Read the model definition and answer for the solid it produces. Units are mm, in the model's axes. Face numbers are marked on the shaded views. Round coordinates to 2 decimals unless told otherwise and drop trailing zeros. Write each loop counter-clockwise with the first axis right and the second up, starting at its lowest first coordinate (ties: lowest second). Pieces come first, ordered by that corner, then holes. Notation, with made-up numbers: (32, 23) -> (38, 23) arc R21 cw to (38, 57) -> close; hole circle Ø11 at (83, -2.5). An arc over 180 degrees is marked (long way). Return JSON: item names as keys, results as strings. Group by question number.
(1) The mould has two halves that part along X. Classify the marked faces 1, 2 and 3: released by +X, released by -X, zero draft, split by the parting line, or undercut.
(2) Straight lines are drawn through the part: line 1 (Z direction, x = -1, y = -0.2); line 2 (X direction, y = -0.75, z = -2.1); line 3 (Z direction, x = 17, y = -0.55). For each, find the intervals that lie inside material, in ascending order.
(3) A cutting plane is placed at B-B on x = 0. Give the vertices of the cut face in (y, z) (3 decimals).
(4) A cutting plane is placed at A-A on y = -1. Give the vertices of the cut face in (x, z), then the cut area to 3 significant figures.
(5) A cutting plane is placed at C-C on x = -12.5. Give the vertices of the cut face in (y, z) (3 decimals), then the cut area to 3 significant figures.
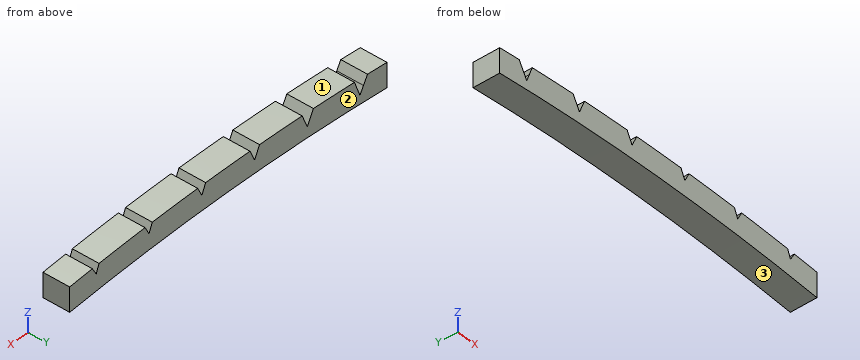
```python
from build123d import *

# Parameters (mm, degrees)
F2_DEPTH = 3.175
F4_DEPTH = 3.176


with BuildPart() as f2:
    # F1 (on Front) → F2 (new body)
    with BuildSketch(Plane.XZ):
        with BuildLine():
            Line((21.4122, -3.8375487704), (21.4122, -0.9419487704))
            ThreePointArc((21.4122, -0.9419487704), (0, 0), (-21.4122, -0.9419487704))
            Line((-21.4122, -0.9419487704), (-21.4122, -3.8375487704))
            ThreePointArc((-21.4122, -3.8375487704), (0, -2.8856456864), (21.4122, -3.8375487704))
        make_face()
    extrude(amount=F2_DEPTH)

    # F3 (on face) → F4 (cut, through all)
    with BuildSketch(Plane.XZ.offset(3.175)):
        with BuildLine():
            Line((-16.877150001, -0.2302185732), (-18.9748496265, -0.3844076014))
            Line((-18.9748496265, -0.3844076014), (-18.2392657349, -1.6819258763))
            ThreePointArc((-18.2392657349, -1.6819258763), (-17.9581295067, -1.0143624708), (-17.3843341446, -1.4564454512))
            ThreePointArc((-17.3843341446, -1.4564454512), (-17.3920934435, -1.5403197391), (-17.4151079687, -1.6213471081))
            Line((-17.4151079687, -1.6213471081), (-16.877150001, -0.2302185732))
        make_face()
        with BuildLine():
            ThreePointArc((-17.4151079687, -1.6213471081), (-17.808018602, -1.9124153497), (-18.2392657349, -1.6819258763))
            Line((-18.2392657349, -1.6819258763), (-17.7632411909, -2.5215997085))
            Line((-17.7632411909, -2.5215997085), (-17.4151079687, -1.6213471081))
        make_face()
        with BuildLine():
            ThreePointArc((-17.3843341446, -1.4564454512), (-17.9581295067, -1.0143624708), (-18.2392657349, -1.6819258763))
            ThreePointArc((-18.2392657349, -1.6819258763), (-17.808018602, -1.9124153497), (-17.4151079687, -1.6213471081))
            ThreePointArc((-17.4151079687, -1.6213471081), (-17.3920934435, -1.5403197391), (-17.3843341446, -1.4564454512))
        make_face()
        Polygon((-11.8018317816, 0.3221485882), (-10.6535149923, -1.8497062999), (-9.7005085696, 0.4146620143), align=None)
        Polygon((-4.6297261067, 0.8171098674), (-3.5456917006, -1.3875339838), (-2.5265922736, 0.8478678732), align=None)
        Polygon((2.5609041822, 1.0761222144), (3.5797209294, -1.1594084921), (4.6640341091, 1.0450982628), align=None)
        Polygon((9.7571629435, 0.9970667736), (10.709883024, -1.2674220323), (11.8584744402, 0.9042876313), align=None)
        Polygon((16.9491408118, 0.681489948), (17.8349422443, -1.6100032173), (19.046820923, 0.5270356622), align=None)
    extrude(amount=-F4_DEPTH, mode=Mode.SUBTRACT)


solid = f2.part
```
Checks:
{
 "1": {"face 1": "released by -X", "face 2": "zero draft", "face 3": "undercut"},
 "2": {"line 1": "z = -2.89 to 0", "line 2": "x = -21.41 to -18, -17.6 to 21.41", "line 3": "z = -3.49 to -0.59"},
 "3": {"outline": "(-3.175, -2.886) -> (0, -2.886) -> (0, 0) -> (-3.175, 0) -> close"},
 "4": {"outline": "(-21.41, -3.84) arc R241.3 cw to (21.41, -3.84) -> (21.41, -0.94) arc R243.84 ccw to (18.36, -0.69) -> (17.83, -1.61) -> (17.45, -0.63) arc R243.84 ccw to (11.24, -0.26) -> (10.71, -1.27) -> (10.27, -0.22) arc R243.84 ccw to (4.13, -0.04) -> (3.58, -1.16) -> (3.06, -0.02) arc R243.84 ccw to (-2.92, -0.02) -> (-3.55, -1.39) -> (-4.21, -0.04) arc R243.84 ccw to (-9.96, -0.2) -> (-10.65, -1.85) -> (-11.49, -0.27) arc R243.84 ccw to (-17.02, -0.59) -> (-17.76, -2.52) -> (-18.78, -0.72) arc R243.84 ccw to (-21.41, -0.94) -> close", "area": "118 mm^2"},
 "5": {"outline": "(-3.175, -3.21) -> (0, -3.21) -> (0, -0.321) -> (-3.175, -0.321) -> close", "area": "9.17 mm^2"}
}
